Check sheet for the modelled part. Datum: model origin and axes. Units: mm. A direction names the side the tool comes from. Round coordinates to 2 decimals unless told otherwise and drop trailing zeros. Order: outer loops, then holes, each group sorted by start corner. A loop starts at its lowest first (then second) coordinate and runs counter-clockwise, first axis right, second up.
```python
from build123d import *

# Parameters (mm, degrees)
SKETCH_W      = 52
SKETCH_H      = 52
SKETCH_R      = 1.8
SKETCH_W_2    = 38
SKETCH_H_2    = 11.5
PAD_DEPTH     = 2
SKETCH001_R   = 2
SKETCH001_R_2 = 3
SKETCH001_R_3 = 1.8
PAD001_DEPTH  = 4.4


with BuildPart() as part:
    # Sketch → Pad (new body)
    with BuildSketch(Plane.XY):
        Rectangle(SKETCH_W, SKETCH_H)
        with Locations((22.25, 22.25)):
            Circle(SKETCH_R, mode=Mode.SUBTRACT)
        with Locations((22.25, -22.25)):
            Circle(SKETCH_R, mode=Mode.SUBTRACT)
        with Locations((-22.25, 22.25)):
            Circle(SKETCH_R, mode=Mode.SUBTRACT)
        with Locations((-22.25, -22.25)):
            Circle(SKETCH_R, mode=Mode.SUBTRACT)
        with Locations((-10.65, 15.5)):
            Circle(SKETCH_R, mode=Mode.SUBTRACT)
        with Locations((10.6, 15.5)):
            Circle(SKETCH_R, mode=Mode.SUBTRACT)
        with Locations((0, -13.25)):
            Rectangle(SKETCH_W_2, SKETCH_H_2, mode=Mode.SUBTRACT)
    extrude(amount=PAD_DEPTH)

    # Sketch001 → Pad001 (new body)
    with BuildSketch(Plane.XY.offset(2)):
        with Locations((0, -5.4)):
            Circle(SKETCH001_R)
        with Locations((-10.65, 15.5)):
            Circle(SKETCH001_R_2)
        with Locations((-10.65, 15.5)):
            Circle(SKETCH001_R_3, mode=Mode.SUBTRACT)
        with Locations((10.6, 15.5)):
            Circle(SKETCH001_R_2)
        with Locations((10.6, 15.5)):
            Circle(SKETCH001_R_3, mode=Mode.SUBTRACT)
    extrude(amount=PAD001_DEPTH)


solid = part.part
```
Item 1: Go/stop test with flat-tipped pins: P1, Ø4.5, axis at x = -10.65, y = 15.5, coming from the +Z side; P2, Ø6, axis at x = 16, y = -5.5, coming from the +Z side. Record where each tip stops, or that it passes through.
Answer:
P1: stops at z = 6.4
P2: stops at z = 2
Item 2: Scan lines: line 1 along Y through (x, z) = (10.6, 1.5); line 2 along Y through (x, z) = (22.25, 1); line 3 along X through (y, z) = (-16, 0.75). Record each from-to range of solid material in increasing order.
Answer:
line 1: y = -26 to -19, -7.5 to 13.7, 17.3 to 26
line 2: y = -26 to -24.05, -20.45 to 20.45, 24.05 to 26
line 3: x = -26 to -19, 19 to 26
Item 3: Sectioned sample at C-C (x = 22.25). Record the cut outline in (y, z).
Answer:
outline: (-26, 0) - (-24.05, 0) - (-24.05, 2) - (-26, 2) - close; (-20.45, 0) - (20.45, 0) - (20.45, 2) - (-20.45, 2) - close; (24.05, 0) - (26, 0) - (26, 2) - (24.05, 2) - close
Item 4: Access from +Z, -Z, +X, -X, +Y, -Y to the whole of each face (thin tool, end or side, straight path). Record for faces 1 (the flat face through (0, 6, 0)), 2 (the flat face through (0, -19, 1)), 3 (the cylindrical face through (-13.031, 13.675, 4.169)).
Answer:
face 1: -Z, +X, -X, +Y, -Y
face 2: +Z, -Z
face 3: +Z
Item 5: Sectioned sample at B-B (y = 15.5). Record the cut outline in (x, z).
Answer:
outline: (-26, 0) - (-12.45, 0) - (-12.45, 6.4) - (-13.65, 6.4) - (-13.65, 2) - (-26, 2) - close; (-8.85, 0) - (8.8, 0) - (8.8, 6.4) - (7.6, 6.4) - (7.6, 2) - (-7.65, 2) - (-7.65, 6.4) - (-8.85, 6.4) - close; (12.4, 0) - (26, 0) - (26, 2) - (13.6, 2) - (13.6, 6.4) - (12.4, 6.4) - close
Item 6: Sectioned sample at D-D (y = -15). Record the cut outline in (x, z), and give its area (3 significant figures).
Answer:
outline: (-26, 0) - (-19, 0) - (-19, 2) - (-26, 2) - close; (19, 0) - (26, 0) - (26, 2) - (19, 2) - close
area: 28.0 mm2
Item 7: Sectioned sample at A-A (z = 3.25). Record the cut outline in (x, y), and give its area (3 significant figures).
Answer:
outline: circle Ø6 at (-10.65, 15.5); circle Ø4 at (0, -5.4); circle Ø6 at (10.6, 15.5); hole circle Ø3.6 at (-10.65, 15.5); hole circle Ø3.6 at (10.6, 15.5)
area: 48.8 mm2
Item 8: Release check for a two-part mould opening along X. For faces 4 (the cylindrical face through (-0.434, -7.352, 4.169)), 5 (the cylindrical face through (23.218, 23.768, 0.986)), 6 (the flat face through (0, 26, 1)) record: released by +X, released by -X, zero draft, split by the parting line, or undercut.
Answer:
face 4: split by the parting line
face 5: undercut
face 6: zero draft
